The model under review builds one solid part; all positions refer to its coordinate system, in mm. Coordinates: 2 decimals unless noted, no trailing zeros. Order: outer loops, then holes, each group sorted by start corner. A loop starts at its lowest first (then second) coordinate and runs counter-clockwise, first axis right, second up. Notation, with made-up numbers: M -38.5,81 L -23.5,81 A25 ccw -23.5,113 Z; hole C 69.5,17 d4. An arc over 180 degrees is marked long. One line per item, written item: value.
```python
from build123d import *

# Parameters (mm, degrees)
BOSS_EXTRUDE1_DEPTH = 1.5875
CUT_EXTRUDE1_REACH  = 222.409
SKETCH3_R           = 14.2875


with BuildPart() as part:
    # Sketch2 → Boss-Extrude1 (new, symmetric)
    with BuildSketch(Plane(origin=(0, 0, 0), x_dir=(1, 0, 0), z_dir=(0, 1, 0))):
        with BuildLine():
            Line((-101.6, 0), (101.6, 0))
            Line((101.6, 0), (101.6, 76.2))
            Line((101.6, 76.2), (9.91703388, 190.80370765))
            ThreePointArc((9.91703388, 190.80370765), (0, 195.570080546), (-9.91703388, 190.80370765))
            Line((-9.91703388, 190.80370765), (-101.6, 76.2))
            Line((-101.6, 76.2), (-101.6, 0))
        make_face()
    extrude(amount=BOSS_EXTRUDE1_DEPTH, both=True)

    # Sketch3 → Cut-Extrude1 (cut, up to next)
    with BuildSketch(Plane(origin=(0, 1.5875, 0), x_dir=(1, 0, 0), z_dir=(0, 1, 0)), mode=Mode.PRIVATE) as cut_extrude1_sk1:
        with Locations(Location((0, 152.375201365, 0), (0, 0, 270))):
            Circle(SKETCH3_R)
    cut_extrude1_tool1 = extrude(cut_extrude1_sk1.sketch, amount=-CUT_EXTRUDE1_REACH, mode=Mode.PRIVATE) & part.part
    add(cut_extrude1_tool1.solids().sort_by_distance((0, 1.5875, -152.375201))[0], mode=Mode.SUBTRACT)


solid = part.part
```
(1) We need section C-C, the plane z = -81. State the section outline as (x, y) points, plus the area to 3 significant figures.
Geometry results:
outline: M -97.76,-1.59 L 97.76,-1.59 L 97.76,1.59 L -97.76,1.59 Z
area: 621 mm2
(2) Insertion check: pin 1 Ø23 at (x, z) = (0, -152.38) entering from -Y; pin 2 Ø1.5 at (y, z) = (-0.5, -124) entering from +X. Each pin has a flat end and moves straight along its axis. Give the tip position at first contact, or say it passes through.
Geometry results:
pin 1: passes through
pin 2: stops at x = 63.96
(3) We need section B-B, the plane x = 0. State the section outline as (y, z) points.
Geometry results:
outline: M -1.59,-195.57 L 1.59,-195.57 L 1.59,-166.66 L -1.59,-166.66 Z; M -1.59,-138.09 L 1.59,-138.09 L 1.59,0 L -1.59,0 Z
(4) We need section D-D, the plane x = -86. State the section outline as (y, z) points.
Geometry results:
outline: M -1.59,-95.7 L 1.59,-95.7 L 1.59,0 L -1.59,0 Z
(5) For L1, parallel to Z at x = 8, y = -0.55; L2, parallel to X at y = 0, z = -152.5; L3, parallel to X at y = -0.75, z = -178.5, list the stretches that pass through material, from the lowest coordinate up.
Geometry results:
L1: z = -192.73 to -164.21, -140.54 to 0
L2: x = -40.56 to -14.29, 14.29 to 40.56
L3: x = -19.76 to 19.76
(6) Mouldability with a two-part tool opening along Z and no side actions: class faces 1 (the flat face through (-1, 1.588, -77)), 2 (the cylindrical face through (-5.472, 0.022, -139.177)), 3 (the flat face through (-55.12, 0.02, -134.3)) as +Z half, -Z half, draft (parallel to the pull), parting line (faces both ways), or undercut.
Geometry results:
face 1: draft
face 2: undercut
face 3: -Z half
(7) We need section A-A, the plane y = -0.25. State the section outline as (x, z) points (1 decimal).
Geometry results:
outline: M -101.6,-76.2 L -9.9,-190.8 A12.7 ccw 9.9,-190.8 L 101.6,-76.2 L 101.6,0 L -101.6,0 Z; hole C 0,-152.4 d28.6
